The model under review builds one solid part; all positions refer to its coordinate system, in mm. Face numbers are marked on the shaded views. A direction names the side the tool comes from. Round coordinates to 2 decimals unless told otherwise and drop trailing zeros. Order: outer loops, then holes, each group sorted by start corner. A loop starts at its lowest first (then second) coordinate and runs counter-clockwise, first axis right, second up. Notation, with made-up numbers: M 14.5,-35.75 L 23.5,-35.75 A6 ccw 23.5,-26.75 Z; hole C 24,29 d11. An arc over 180 degrees is marked long. Answer as a JSON object with one key per item and string values. Group by question number.
1. Add section B-B on z = 2.5. State the section outline as (x, y) points (3 decimals).
2. To check wall thickness, follow probe 1 along X at (y, z) = (19, 6.25); probe 2 along X at (y, z) = (12.5, 10.5); probe 3 along Y at (x, z) = (17, 5.5). State the ranges of each line that lie inside material, in increasing order. Write a range as [from, to].
3. Add section D-D on y = 20.5. State the section outline as (x, z) points.
4. Add section C-C on x = -4.5. State the section outline as (y, z) points.
5. Add section A-A on z = 0.75. State the section outline as (x, y) points (3 decimals).
6. Mouldability with a two-part tool opening along X and no side actions: class the marked faces 1, 2 and 3 as released by +X, released by -X, zero draft, split by the parting line, or undercut.
7. Machinability: for the marked faces 4, 5 and 6, which of the approach directions +Z, -Z, +X, -X, +Y, -Y give a long, thin tool a straight path to every point of the face, cutting with its end or side? Answer none if there is none.
8. Clearance check with flat-ended pins moving along their axes: P1, Ø1.5, axis at x = 9.5, y = 20.5, coming from the -Z side; P2, Ø6, axis at x = 2.73, y = 14.92, coming from the -Z side; P3, Ø3, axis at x = -5.24, y = 14.92, coming from the +Z side; P4, Ø0.8, axis at x = 2.5, y = 20, coming from the -Z side. State where each tip first meets the part, or that it passes through.
```python
from build123d import *

# Parameters (mm, degrees)
F0_W     = 31.77
F0_H     = 15.8
F0_R     = 3.215
F0_R_2   = 2.325
F1_DEPTH = 9.53
F2_DEPTH = 8.39
F3_DEPTH = 1.17
F4_R     = 2.44
F5_DEPTH = 1.48


with BuildPart() as f1:
    # F0 (on Top) → F1 (new body)
    with BuildSketch(Plane.XY):
        with Locations((2.730887816, 14.921668646)):
            Rectangle(F0_W, F0_H)
        Polygon((2.360887816, 8.191668646), (-11.984112184, 8.191668646), (-11.984112184, 21.651668646), (2.360887816, 21.651668646), (3.100887816, 21.651668646), (17.445887816, 21.651668646), (17.445887816, 8.191668646), (3.100887816, 8.191668646), align=None, mode=Mode.SUBTRACT)
        with BuildLine():
            Line((-11.984112184, 21.651668646), (-11.984112184, 8.191668646))
            Line((-11.984112184, 8.191668646), (2.360887816, 8.191668646))
            Line((2.360887816, 8.191668646), (2.360887816, 11.7230304386))
            ThreePointArc((2.360887816, 11.7230304386), (-0.484112184, 14.916668646), (2.360887816, 18.1103068535))
            Line((2.360887816, 18.1103068535), (2.360887816, 21.651668646))
            Line((2.360887816, 21.651668646), (-11.984112184, 21.651668646))
        make_face()
        with Locations((-5.239112184, 14.916668646)):
            Circle(F0_R, mode=Mode.SUBTRACT)
        with BuildLine():
            Line((3.100887816, 11.7230304386), (3.100887816, 8.191668646))
            Line((3.100887816, 8.191668646), (17.445887816, 8.191668646))
            Line((17.445887816, 8.191668646), (17.445887816, 21.651668646))
            Line((17.445887816, 21.651668646), (3.100887816, 21.651668646))
            Line((3.100887816, 21.651668646), (3.100887816, 18.1103068535))
            ThreePointArc((3.100887816, 18.1103068535), (5.1314893031, 17.0552049445), (5.945887816, 14.916668646))
            ThreePointArc((5.945887816, 14.916668646), (5.1314893031, 12.7781323475), (3.100887816, 11.7230304386))
        make_face()
        with Locations((10.700887816, 14.916668646)):
            Circle(F0_R, mode=Mode.SUBTRACT)
        with BuildLine():
            ThreePointArc((2.360887816, 18.1103068535), (-0.484112184, 14.916668646), (2.360887816, 11.7230304386))
            ThreePointArc((2.360887816, 11.7230304386), (2.730887816, 11.701668646), (3.100887816, 11.7230304386))
            ThreePointArc((3.100887816, 11.7230304386), (5.1314893031, 12.7781323475), (5.945887816, 14.916668646))
            ThreePointArc((5.945887816, 14.916668646), (5.1314893031, 17.0552049445), (3.100887816, 18.1103068535))
            ThreePointArc((3.100887816, 18.1103068535), (2.730887816, 18.131668646), (2.360887816, 18.1103068535))
        make_face()
        with Locations((2.730887816, 14.916668646)):
            Circle(F0_R_2, mode=Mode.SUBTRACT)
        with Locations((10.700887816, 14.916668646)):
            Circle(F0_R)
        with Locations((10.700887816, 14.916668646)):
            Circle(F0_R_2, mode=Mode.SUBTRACT)
        with Locations((-5.239112184, 14.916668646)):
            Circle(F0_R)
        with Locations((-5.239112184, 14.916668646)):
            Circle(F0_R_2, mode=Mode.SUBTRACT)
        with Locations((10.700887816, 14.916668646)):
            Circle(F0_R_2)
        with Locations((-5.239112184, 14.916668646)):
            Circle(F0_R_2)
        with Locations((2.730887816, 14.916668646)):
            Circle(F0_R_2)
        with BuildLine():
            Line((3.100887816, 21.651668646), (2.360887816, 21.651668646))
            Line((2.360887816, 21.651668646), (2.360887816, 18.1103068535))
            ThreePointArc((2.360887816, 18.1103068535), (2.730887816, 18.131668646), (3.100887816, 18.1103068535))
            Line((3.100887816, 18.1103068535), (3.100887816, 21.651668646))
        make_face()
        with BuildLine():
            Line((2.360887816, 11.7230304386), (2.360887816, 8.191668646))
            Line((2.360887816, 8.191668646), (3.100887816, 8.191668646))
            Line((3.100887816, 8.191668646), (3.100887816, 11.7230304386))
            ThreePointArc((3.100887816, 11.7230304386), (2.730887816, 11.701668646), (2.360887816, 11.7230304386))
        make_face()
    extrude(amount=F1_DEPTH)

    # F0 (on Top) → F2 (cut)
    with BuildSketch(Plane.XY):
        with BuildLine():
            Line((-11.984112184, 21.651668646), (-11.984112184, 8.191668646))
            Line((-11.984112184, 8.191668646), (2.360887816, 8.191668646))
            Line((2.360887816, 8.191668646), (2.360887816, 11.7230304386))
            ThreePointArc((2.360887816, 11.7230304386), (-0.484112184, 14.916668646), (2.360887816, 18.1103068535))
            Line((2.360887816, 18.1103068535), (2.360887816, 21.651668646))
            Line((2.360887816, 21.651668646), (-11.984112184, 21.651668646))
        make_face()
        with Locations((-5.239112184, 14.916668646)):
            Circle(F0_R, mode=Mode.SUBTRACT)
        with BuildLine():
            Line((3.100887816, 11.7230304386), (3.100887816, 8.191668646))
            Line((3.100887816, 8.191668646), (17.445887816, 8.191668646))
            Line((17.445887816, 8.191668646), (17.445887816, 21.651668646))
            Line((17.445887816, 21.651668646), (3.100887816, 21.651668646))
            Line((3.100887816, 21.651668646), (3.100887816, 18.1103068535))
            ThreePointArc((3.100887816, 18.1103068535), (5.1314893031, 17.0552049445), (5.945887816, 14.916668646))
            ThreePointArc((5.945887816, 14.916668646), (5.1314893031, 12.7781323475), (3.100887816, 11.7230304386))
        make_face()
        with Locations((10.700887816, 14.916668646)):
            Circle(F0_R, mode=Mode.SUBTRACT)
        with Locations((10.700887816, 14.916668646)):
            Circle(F0_R_2)
        with Locations((2.730887816, 14.916668646)):
            Circle(F0_R_2)
        with Locations((-5.239112184, 14.916668646)):
            Circle(F0_R_2)
    extrude(amount=F2_DEPTH, mode=Mode.SUBTRACT)

    # F0 (on Top) → F3 (cut)
    with BuildSketch(Plane.XY):
        with BuildLine():
            Line((2.360887816, 11.7230304386), (2.360887816, 8.191668646))
            Line((2.360887816, 8.191668646), (3.100887816, 8.191668646))
            Line((3.100887816, 8.191668646), (3.100887816, 11.7230304386))
            ThreePointArc((3.100887816, 11.7230304386), (2.730887816, 11.701668646), (2.360887816, 11.7230304386))
        make_face()
        with BuildLine():
            Line((3.100887816, 21.651668646), (2.360887816, 21.651668646))
            Line((2.360887816, 21.651668646), (2.360887816, 18.1103068535))
            ThreePointArc((2.360887816, 18.1103068535), (2.730887816, 18.131668646), (3.100887816, 18.1103068535))
            Line((3.100887816, 18.1103068535), (3.100887816, 21.651668646))
        make_face()
    extrude(amount=F3_DEPTH, mode=Mode.SUBTRACT)

    # F4 (on face) → F5 (join)
    with BuildSketch(Plane.XY.offset(9.53)):
        with Locations((-9.374112184, 19.101668646)):
            Circle(F4_R)
        with Locations((-9.374112184, 10.741668646)):
            Circle(F4_R)
        with Locations((-1.304112184, 19.101668646)):
            Circle(F4_R)
        with Locations((-1.304112184, 10.741668646)):
            Circle(F4_R)
        with Locations((6.765887816, 19.101668646)):
            Circle(F4_R)
        with Locations((6.765887816, 10.741668646)):
            Circle(F4_R)
        with Locations((14.835887816, 19.101668646)):
            Circle(F4_R)
        with Locations((14.835887816, 10.741668646)):
            Circle(F4_R)
    extrude(amount=F5_DEPTH)


solid = f1.part
```
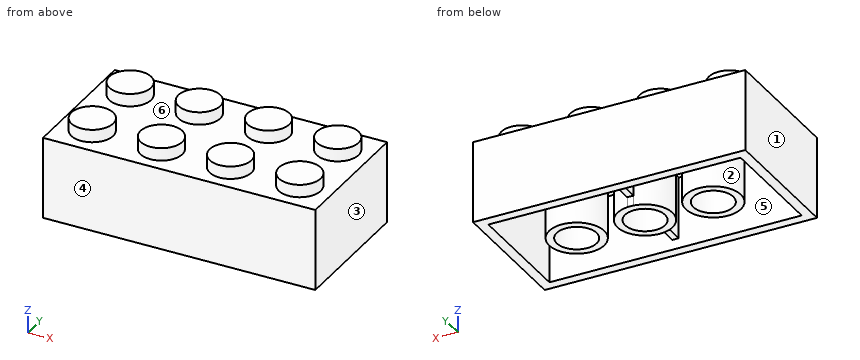
Recorded:
{
 "1": {"outline": "M -13.154,7.022 L 18.616,7.022 L 18.616,22.822 L -13.154,22.822 Z; C -5.239,14.917 d6.43; C 10.701,14.917 d6.43; hole M -11.984,8.192 L 2.361,8.192 L 2.361,11.723 A3.215 cw 2.361,18.11 L 2.361,21.652 L -11.984,21.652 Z; hole C -5.239,14.917 d4.65; hole C 2.731,14.917 d4.65; hole M 3.101,8.192 L 17.446,8.192 L 17.446,21.652 L 3.101,21.652 L 3.101,18.11 A3.215 cw 3.101,11.723 Z; hole C 10.701,14.917 d4.65"},
 "2": {"probe 1": "x = [-13.15, -11.98], [2.36, 3.1], [17.45, 18.62]", "probe 2": "x = [-11.07, -7.68], [-3, 0.39], [5.07, 8.46], [13.14, 16.53]", "probe 3": "y = [7.02, 8.19], [21.65, 22.82]"},
 "3": {"outline": "M -13.15,0 L -11.98,0 L -11.98,8.39 L 2.36,8.39 L 2.36,1.17 L 3.1,1.17 L 3.1,8.39 L 17.45,8.39 L 17.45,0 L 18.62,0 L 18.62,9.53 L 16.84,9.53 L 16.84,11.01 L 12.84,11.01 L 12.84,9.53 L 8.77,9.53 L 8.77,11.01 L 4.77,11.01 L 4.77,9.53 L 0.7,9.53 L 0.7,11.01 L -3.3,11.01 L -3.3,9.53 L -7.37,9.53 L -7.37,11.01 L -11.37,11.01 L -11.37,9.53 L -13.15,9.53 Z"},
 "4": {"outline": "M 7.02,0 L 8.19,0 L 8.19,8.39 L 11.79,8.39 L 11.79,0 L 12.71,0 L 12.71,8.39 L 17.12,8.39 L 17.12,0 L 18.05,0 L 18.05,8.39 L 21.65,8.39 L 21.65,0 L 22.82,0 L 22.82,9.53 L 7.02,9.53 Z"},
 "5": {"outline": "M -13.154,7.022 L 18.616,7.022 L 18.616,22.822 L -13.154,22.822 Z; C -5.239,14.917 d6.43; C 2.731,14.917 d6.43; C 10.701,14.917 d6.43; hole M -11.984,8.192 L 17.446,8.192 L 17.446,21.652 L -11.984,21.652 Z; hole C -5.239,14.917 d4.65; hole C 2.731,14.917 d4.65; hole C 10.701,14.917 d4.65"},
 "6": {"face 1": "released by -X", "face 2": "undercut", "face 3": "released by +X"},
 "7": {"face 4": "+Z, -Z, +X, -X, -Y", "face 5": "-Z", "face 6": "+Z"},
 "8": {"P1": "stops at z = 8.39", "P2": "stops at z = 0", "P3": "stops at z = 9.53", "P4": "stops at z = 1.17"}
}
